Source: CAD feature listing. Evaluate the final solid. Frame: model axes, mm. A direction names the side the tool comes from. Coordinates: 2 decimals unless noted, no trailing zeros. Order: outer loops, then holes, each group sorted by start corner. A loop starts at its lowest first (then second) coordinate and runs counter-clockwise, first axis right, second up. Notation, with made-up numbers: (53.25, 62) -> (107.25, 62) arc R23 ccw to (107.25, 101) -> close; hole circle Ø3 at (-36.5, -5.5). An arc over 180 degrees is marked (long way). Put each result on its own line as item: value.
from build123d import *

# Parameters (mm, degrees)
F0_W     = 2
F0_H     = 1
F1_DEPTH = 100


with BuildPart() as f1:
    # F0 (on Front) → F1 (new body)
    with BuildSketch(Plane.XZ):
        with BuildLine():
            Line((37.4444444444, 14.6527777778), (-35.5555555556, 14.6527777778))
            ThreePointArc((-35.5555555556, 14.6527777778), (-35.9091089461, 14.5063311684), (-36.0555555556, 14.1527777778))
            Line((-36.0555555556, 14.1527777778), (-36.0555555556, -13.8472222222))
            ThreePointArc((-36.0555555556, -13.8472222222), (-35.9091089461, -14.2007756128), (-35.5555555556, -14.3472222222))
            Line((-35.5555555556, -14.3472222222), (37.4444444444, -14.3472222222))
            ThreePointArc((37.4444444444, -14.3472222222), (37.797997835, -14.2007756128), (37.9444444444, -13.8472222222))
            Line((37.9444444444, -13.8472222222), (37.9444444444, 14.1527777778))
            ThreePointArc((37.9444444444, 14.1527777778), (37.797997835, 14.5063311684), (37.4444444444, 14.6527777778))
        make_face()
        Polygon((-31.0555555556, 12.6527777778), (32.9444444444, 12.6527777778), (34.9444444444, 12.6527777778), (35.9444444444, 12.6527777778), (35.9444444444, 11.6527777778), (35.9444444444, 9.6527777778), (35.9444444444, -2.3472222222), (35.9444444444, -3.3472222222), (35.9444444444, -5.3472222222), (35.9444444444, -6.3472222222), (35.9444444444, -8.3472222222), (35.9444444444, -9.3472222222), (35.9444444444, -11.3472222222), (35.9444444444, -12.3472222222), (34.9444444444, -12.3472222222), (32.9444444444, -12.3472222222), (-31.0555555556, -12.3472222222), (-33.0555555556, -12.3472222222), (-34.0555555556, -12.3472222222), (-34.0555555556, -11.3472222222), (-34.0555555556, -9.3472222222), (-34.0555555556, -8.3472222222), (-34.0555555556, -6.3472222222), (-34.0555555556, -5.3472222222), (-34.0555555556, -3.3472222222), (-34.0555555556, -2.3472222222), (-34.0555555556, 9.6527777778), (-34.0555555556, 11.6527777778), (-34.0555555556, 12.6527777778), (-33.0555555206, 12.6527777778), align=None, mode=Mode.SUBTRACT)
        with BuildLine():
            Line((34.9444444444, 12.6527777778), (32.9444444444, 12.6527777778))
            Line((32.9444444444, 12.6527777778), (32.9444444444, 11.6527777778))
            ThreePointArc((32.9444444444, 11.6527777778), (33.5302308821, 10.2385642154), (34.9444444444, 9.6527777778))
            Line((34.9444444444, 9.6527777778), (35.9444444444, 9.6527777778))
            Line((35.9444444444, 9.6527777778), (35.9444444444, 11.6527777778))
            ThreePointArc((35.9444444444, 11.6527777778), (34.2373376633, 10.9456709966), (34.9444444444, 12.6527777778))
        make_face()
        with BuildLine():
            Line((35.9444444444, -11.3472222222), (35.9444444444, -9.3472222222))
            Line((35.9444444444, -9.3472222222), (34.9444444444, -9.3472222222))
            ThreePointArc((34.9444444444, -9.3472222222), (34.4268063542, -9.4153705696), (33.9444444444, -9.6151714147))
            ThreePointArc((33.9444444444, -9.6151714147), (33.2123936369, -10.3472222222), (32.9444444444, -11.3472222222))
            Line((32.9444444444, -11.3472222222), (32.9444444444, -12.3472222222))
            Line((32.9444444444, -12.3472222222), (34.9444444444, -12.3472222222))
            ThreePointArc((34.9444444444, -12.3472222222), (34.2373376633, -10.640115441), (35.9444444444, -11.3472222222))
        make_face()
        with BuildLine():
            Line((-31.0555555556, 11.6527777778), (-31.0555555556, 12.6527777778))
            Line((-31.0555555556, 12.6527777778), (-33.0555555206, 12.6527777778))
            ThreePointArc((-33.0555555206, 12.6527777778), (-32.348448762, 12.3598845466), (-32.0555555556, 11.6527777778))
            ThreePointArc((-32.0555555556, 11.6527777778), (-33.0555555556, 10.6527777778), (-34.0555555556, 11.6527777778))
            Line((-34.0555555556, 11.6527777778), (-34.0555555556, 9.6527777778))
            Line((-34.0555555556, 9.6527777778), (-33.0555555556, 9.6527777778))
            ThreePointArc((-33.0555555556, 9.6527777778), (-31.6413419932, 10.2385642154), (-31.0555555556, 11.6527777778))
        make_face()
        with BuildLine():
            Line((-33.0555555556, -9.3472222222), (-34.0555555556, -9.3472222222))
            Line((-34.0555555556, -9.3472222222), (-34.0555555556, -11.3472222222))
            ThreePointArc((-34.0555555556, -11.3472222222), (-33.0555555556, -10.3472222222), (-32.0555555556, -11.3472222222))
            ThreePointArc((-32.0555555556, -11.3472222222), (-32.3484487744, -12.0543290034), (-33.0555555556, -12.3472222222))
            Line((-33.0555555556, -12.3472222222), (-31.0555555556, -12.3472222222))
            Line((-31.0555555556, -12.3472222222), (-31.0555555556, -11.3472222222))
            ThreePointArc((-31.0555555556, -11.3472222222), (-31.323504748, -10.3472222222), (-32.0555555556, -9.6151714147))
            ThreePointArc((-32.0555555556, -9.6151714147), (-32.5379174654, -9.4153705696), (-33.0555555556, -9.3472222222))
        make_face()
        with BuildLine():
            Line((35.9444444444, -9.3472222222), (35.9444444444, -8.3472222222))
            Line((35.9444444444, -8.3472222222), (33.9444444444, -8.3472222222))
            Line((33.9444444444, -8.3472222222), (33.9444444444, -9.6151714147))
            ThreePointArc((33.9444444444, -9.6151714147), (34.4268063542, -9.4153705696), (34.9444444444, -9.3472222222))
            Line((34.9444444444, -9.3472222222), (35.9444444444, -9.3472222222))
        make_face()
        with BuildLine():
            Line((-32.0555555556, -8.3472222222), (-34.0555555556, -8.3472222222))
            Line((-34.0555555556, -8.3472222222), (-34.0555555556, -9.3472222222))
            Line((-34.0555555556, -9.3472222222), (-33.0555555556, -9.3472222222))
            ThreePointArc((-33.0555555556, -9.3472222222), (-32.5379174654, -9.4153705696), (-32.0555555556, -9.6151714147))
            Line((-32.0555555556, -9.6151714147), (-32.0555555556, -8.3472222222))
        make_face()
        with Locations((34.9444444444, -5.8472222222)):
            Rectangle(F0_W, F0_H)
        with Locations((-33.0555555556, -5.8472222222)):
            Rectangle(F0_W, F0_H)
        with Locations((-33.0555555556, -2.8472222222)):
            Rectangle(F0_W, F0_H)
        with Locations((34.9444444444, -2.8472222222)):
            Rectangle(F0_W, F0_H)
        with BuildLine():
            Line((35.9444444444, 12.6527777778), (34.9444444444, 12.6527777778))
            ThreePointArc((34.9444444444, 12.6527777778), (35.6515512256, 12.359884559), (35.9444444444, 11.6527777778))
            Line((35.9444444444, 11.6527777778), (35.9444444444, 12.6527777778))
        make_face()
        with BuildLine():
            Line((35.9444444444, -12.3472222222), (35.9444444444, -11.3472222222))
            ThreePointArc((35.9444444444, -11.3472222222), (35.6515512256, -12.0543290034), (34.9444444444, -12.3472222222))
            Line((34.9444444444, -12.3472222222), (35.9444444444, -12.3472222222))
        make_face()
        with BuildLine():
            ThreePointArc((-34.0555555556, 11.6527777778), (-33.7626623244, 12.3598845713), (-33.0555555206, 12.6527777778))
            Line((-33.0555555206, 12.6527777778), (-34.0555555556, 12.6527777778))
            Line((-34.0555555556, 12.6527777778), (-34.0555555556, 11.6527777778))
        make_face()
        with BuildLine():
            ThreePointArc((-33.0555555556, -12.3472222222), (-33.7626623367, -12.0543290034), (-34.0555555556, -11.3472222222))
            Line((-34.0555555556, -11.3472222222), (-34.0555555556, -12.3472222222))
            Line((-34.0555555556, -12.3472222222), (-33.0555555556, -12.3472222222))
        make_face()
    extrude(amount=F1_DEPTH)


solid = f1.part
1. Pull-direction query (X, two-part tool) for faces 3 (the flat face through (-36.056, -49, 0)), 4 (the flat face through (1, -49, 14.653)), 5 (the flat face through (35, -49, -8.347)); classes: pulls with the +X half, pulls with the -X half, needs draft (parallel to the pull), parting line crosses it, or undercut.
Numbers:
face 3: pulls with the -X half
face 4: needs draft
face 5: undercut
2. Cut plane C-C on y = -7.5. Count the separate pieces of the cut face and the enclosed holes in it, plus the area to 3 significant figures.
Numbers:
separate pieces: 1
enclosed holes: 5
area: 428 mm2
3. Ray query, line 1 along X through (y, z) = (-28.5, -5.5); line 2 along Z through (x, y) = (-6.5, -40.5); line 3 along X through (y, z) = (-34, -0.5). Return the intervals inside material, ascending.
Numbers:
line 1: x = -36.06 to -32.06, 33.94 to 37.94
line 2: z = -14.35 to -12.35, 12.65 to 14.65
line 3: x = -36.06 to -34.06, 35.94 to 37.94
4. Cut plane B-B on z = 5.5. Output: boundary loops of the cut face in (x, y).
Numbers:
outline: (-36.06, -100) -> (-34.06, -100) -> (-34.06, 0) -> (-36.06, 0) -> close; (35.94, -100) -> (37.94, -100) -> (37.94, 0) -> (35.94, 0) -> close
5. Set-up query: faces 1 (the flat face through (-33, -49, -5.347)), 2 (the flat face through (0, -49, -14.347)). Return all of +Z, -Z, +X, -X, +Y, -Y with unobstructed straight access to the full face (end or side cutting, diameter ignored); none if empty.
Numbers:
face 1: +Y, -Y
face 2: -Z, +X, -X, +Y, -Y
6. Cut plane A-A on x = -9. Output: boundary loops of the cut face in (y, z).
Numbers:
outline: (-100, -14.35) -> (0, -14.35) -> (0, -12.35) -> (-100, -12.35) -> close; (-100, 12.65) -> (0, 12.65) -> (0, 14.65) -> (-100, 14.65) -> close
7. First-contact query: pin 1 (12 mm diameter, centred on x = -7, z = -10.5, fed in from -Y). Flat tip, straight axial feed; report the tip coordinate or a pass-through.
Numbers:
pin 1: stops at y = -100
